```python
from build123d import *

# Parameters (mm, degrees)
SKETCH1_W                      = 14
SKETCH1_H                      = 2
CUT_EXTRUDE1_REACH             = 61.5
SKETCH1_3_R                    = 2.5
CUT_EXTRUDE1_DIRECTION_2_REACH = 61.5


with BuildPart() as part:
    # Sketch1 → Revolve1 (revolve)
    with BuildSketch(Plane.XY):
        with Locations((7, 51.5)):
            Rectangle(SKETCH1_W, SKETCH1_H)
        with BuildLine():
            ThreePointArc((0, 52.5), (7, 59.5), (14, 52.5))
            Line((14, 52.5), (0, 52.5))
        make_face()
    revolve(axis=Axis((0, 0, 0), (1, 0, 0)))

    # Sketch1<3> → Cut-Extrude1 (cut, up to next)
    with BuildSketch(Plane.XY, mode=Mode.PRIVATE) as cut_extrude1_sk1:
        with Locations((7, 0)):
            Circle(SKETCH1_3_R)
    cut_extrude1_tool1 = extrude(cut_extrude1_sk1.sketch, amount=-CUT_EXTRUDE1_REACH, mode=Mode.PRIVATE) & part.part
    add(cut_extrude1_tool1.solids().sort_by_distance((7, 0, 0))[0], mode=Mode.SUBTRACT)

    # Sketch1<3> → Cut-Extrude1 direction 2 (cut, up to next)
    with BuildSketch(Plane.XY, mode=Mode.PRIVATE) as cut_extrude1_direction_2_sk1:
        with Locations((7, 0)):
            Circle(SKETCH1_3_R)
    cut_extrude1_direction_2_tool1 = extrude(cut_extrude1_direction_2_sk1.sketch, amount=CUT_EXTRUDE1_DIRECTION_2_REACH, mode=Mode.PRIVATE) & part.part
    add(cut_extrude1_direction_2_tool1.solids().sort_by_distance((7, 0, 0))[0], mode=Mode.SUBTRACT)


solid = part.part
```
Geometry check sheet. Reference: the model listing, model coordinates, mm. Round coordinates to 2 decimals unless told otherwise and drop trailing zeros. Loops run counter-clockwise (first coordinate to the right, second up) from the corner with the lowest first, then second, coordinate; pieces in that order, holes last. Notation, with made-up numbers: M 12,-27.5 L 20,-27.5 A20 ccw 20,9.5 Z; hole C 80,9.5 d3. An arc over 180 degrees is marked long. Return JSON: item names as keys, results as strings. Group by question number.
(1) Section check C-C, the plane y = 0. Enter the section's corners in (x, z), and give its area (3 significant figures).
(2) Scan lines: line 1 along Z through (x, y) = (12, -31.5); line 2 along Y through (x, z) = (12.25, -31); line 3 along Y through (x, z) = (5.5, -31). Record each from-to range of solid material in increasing order. Write a range as [from, to].
(3) Go/stop test with flat-tipped pins: pin 1 (5 mm diameter, centred on x = 6, z = -21.5, fed in from +Y); pin 2 (4 mm diameter, centred on x = 5.5, z = 5.5, fed in from +Y); pin 3 (5 mm diameter, centred on x = 12.5, z = -31, fed in from +Y). Record where each tip stops, or that it passes through.
(4) Section check A-A, the plane z = 0. Enter the section's corners in (x, y), and give its area (3 significant figures).
(5) Section check B-B, the plane x = 7. Enter the section's corners in (y, z), and give its area (3 significant figures).
(6) Mould release check, pull along Y, two halves, no side actions. Record for faces 1 (the face through (9.385, 0.751, 54.88)), 2 (the face through (9.385, 0.751, -54.88)), 3 (the face through (0, 27, 43)): pulls with the +Y half, pulls with the -Y half, needs draft (parallel to the pull), parting line crosses it, or undercut.
Data:
{
 "1": {"outline": "M 0,-52.5 A7 ccw 4.5,-59.04 L 4.5,-50.5 L 0,-50.5 Z; M 0,50.5 L 4.5,50.5 L 4.5,59.04 A7 ccw 0,52.5 Z; M 9.5,-59.04 A7 ccw 14,-52.5 L 14,-50.5 L 9.5,-50.5 Z; M 9.5,50.5 L 14,50.5 L 14,52.5 A7 ccw 9.5,59.04 Z", "area": "121 mm²"},
 "2": {"line 1": "[-47.98, -39.47], [39.47, 47.98]", "line 2": "[-47.99, -39.87], [39.87, 47.99]", "line 3": "[-50.6, -39.87], [39.87, 50.6]"},
 "3": {"pin 1": "y = 56.35", "pin 2": "y = 59.37", "pin 3": "y = 50.59"},
 "4": {"outline": "M 0,-52.5 A7 ccw 14,-52.5 L 14,-50.5 L 0,-50.5 Z; M 0,50.5 L 14,50.5 L 14,52.5 A7 ccw 0,52.5 Z", "area": "210 mm²"},
 "5": {"outline": "M -2.5,-59.45 L -2.5,-50.44 A50.5 cw -2.5,50.44 L -2.5,59.45 A59.5 ccw Z; M 2.5,-59.45 A59.5 ccw 2.5,59.45 L 2.5,50.44 A50.5 cw 2.5,-50.44 Z", "area": "3,020 mm²"},
 "6": {"face 1": "undercut", "face 2": "undercut", "face 3": "needs draft"}
}
